Autodesk Inventor part; units mm, degrees
ref_plane "YZ Plane" through (0, 0, 0) normal (1, 0, 0) x (0, 1, 0)
ref_plane "XZ Plane" through (0, 0, 0) normal (0, 1, 0) x (-1, 0, 0)
ref_plane "XY Plane" through (0, 0, 0) normal (0, 0, 1) x (1, 0, 0)
sketch "Náčrt1" plane through (0, 0, 0) normal (0, 0, 1) x (1, 0, 0)
  line L0 (-4.9375, 15) -> (4.9375, 15)
  line L1 (4.9375, 15) -> (4.9375, -15)
  line L2 (4.9375, -15) -> (-4.9375, -15)
  line L3 (-4.9375, -15) -> (-4.9375, 15)
  line L4 (-4.9375, 15) -> (4.9375, -15) construction
  line L5 (4.9375, 15) -> (-4.9375, -15) construction
  circle A0 centre (0, 10.0625) radius 1.5
  circle A1 centre (0, -10.0625) radius 1.5
  line L6 (-4.9375, 0) -> (4.9375, 0)
  point P0 (0, 0)
  point P1 (0, 15)
  dimension "d0" = 30
  dimension "d1" = 9.875
  dimension "d2" = 3
  dimension "d4" = 4.9375
extrude "Vysunutí1" add sketch "Náčrt1" along normal blind 10
sketch "Náčrt2" plane through (4.9375, -15, 0) normal (1, 0, 0) x (0, 0, -1)
  line L0 (0, 0) -> (0, 30)
  line L1 (0, 10) -> (-3.3166, 10)
  arc A0 (-3.3166, 20) -> (-3.3166, 10) centre (0, 15) ccw
  line L2 (-3.3166, 20) -> (0, 20)
  line L3 (0, 9.875) -> (-3.3541, 9.875)
  arc A1 (-3.3541, 20.125) -> (-3.3541, 9.875) centre (0, 15) ccw
  line L4 (-3.3541, 20.125) -> (0, 20.125)
  line L5 (0, 30) -> (-10, 30)
  line L6 (0, 6.875) -> (-4.1533, 6.875) construction
  arc A2 (-4.1533, 23.125) -> (-4.1533, 6.875) centre (0, 15) ccw construction
  line L7 (-4.1533, 23.125) -> (0, 23.125) construction
  line L8 (0, 0) -> (-10, 0)
  line L9 (-7, 0) -> (-7, 9.1463)
  line L10 (-7, 9.1463) -> (-9, 13.4948)
  line L11 (-9, 16.5052) -> (-7, 20.8537)
  line L12 (-7, 20.8537) -> (-7, 30)
  line L13 (-9, 13.4948) -> (-9, 16.5052)
  line L14 (-10, 0) -> (-10, 30)
  point P0 (0, 15)
  point P1 (0, 9.875)
  point P2 (-9, 15)
  point P3 (-10, 15)
  dimension "d7" = 6
  dimension "d8" = 10
  dimension "d9" = 0.125
  dimension "d16" = 3
  dimension "d17" = 3
  dimension "d18" = 3
  dimension "d19" = 1
extrude "Vysunutí2" cut sketch "Náčrt2" against normal through all contours L3 A1 L4 L0 L2 A0 L1 | L8 L14 L5 L12 L11 L13 L10 L9 | L1 A0 L2 L0
fillet "Zaoblení1" radius 2 4 edges at (0, -1.5052, 9) (0, 1.5052, 9) (0, 5.8537, 7) (0, -5.8537, 7)
fillet "Zaoblení2" radius 0.25 20 edges at (0, -15, 7) (0, 15, 7) (4.9375, -5.8638, 7.0463) (4.9375, -3.6794, 8) (4.9375, -1.4951, 8.9537) (4.9375, 0, 9) (4.9375, 1.4951, 8.9537) (4.9375, 3.6794, 8) (4.9375, 5.8638, 7.0463) (4.9375, 10.6458, 7) (4.9375, -10.6458, 7) (-4.9375, -5.8638, 7.0463) (-4.9375, -3.6794, 8) (-4.9375, -1.4951, 8.9537) (-4.9375, 0, 9) (-4.9375, 1.4951, 8.9537) (-4.9375, 3.6794, 8) (-4.9375, 5.8638, 7.0463) (-4.9375, 10.6458, 7) (-4.9375, -10.6458, 7)
sketch "Náčrt3" plane through (0, 0, 0) normal (0, 0, -1) x (-1, 0, 0)
  line L0 (4.9375, -5.125) -> (-4.9375, -5.125)
  line L1 (-4.9375, -15) -> (-4.9375, -5.125)
  line L2 (4.9375, -15) -> (-4.9375, -15)
  line L3 (4.9375, -5.125) -> (4.9375, -15)
  circle A0 centre (0, -10.0625) radius 1.5
  line L4 (-4.9375, 5.125) -> (4.9375, 5.125)
  line L5 (4.9375, 15) -> (4.9375, 5.125)
  line L6 (-4.9375, 15) -> (4.9375, 15)
  line L7 (-4.9375, 5.125) -> (-4.9375, 15)
  circle A1 centre (0, 10.0625) radius 1.5
  point P0 (0, 0)
extrude "Vysunutí3" cut sketch "Náčrt3" against normal blind 1
chamfer "Zkosení1" distance 0.25 angle 45 6 edges at (4.9375, -5.125, 2.1771) (4.9375, 0, 6.125) (4.9375, 5.125, 2.1771) (-4.9375, -5.125, 2.1771) (-4.9375, 0, 6.125) (-4.9375, 5.125, 2.1771)
fillet "Zaoblení3" radius 0.5 8 edges at (4.8643, -14.9268, 6.9268) (4.9375, -15, 3.875) (-4.8643, -14.9268, 6.9268) (-4.9375, -15, 3.875) (-4.8643, 14.9268, 6.9268) (-4.9375, 15, 3.875) (4.8643, 14.9268, 6.9268) (4.9375, 15, 3.875)
sketch "Náčrt4" plane through (-4.6875, 6.2916, 7) normal (0, 0, 1) x (1, 0, 0)
  circle A0 centre (4.6875, 3.7709) radius 1.5
  point P0 (4.6875, -6.2916)
hole "Díra1" at (0, 10.0625, 7) direction (0, 0, -1) diameter 3.5 end through all countersink diameter 7 countersink angle 90
sketch "Náčrt5" plane through (-4.6875, -6.2916, 7) normal (0, 0, 1) x (1, 0, 0)
  circle A0 centre (4.6875, -3.7709) radius 1.5
  point P0 (4.6875, 6.2916)
hole "Díra2" at (0, -10.0625, 7) direction (0, 0, -1) diameter 3.5 end through all countersink diameter 7 countersink angle 90
properties part number "Objímka motoru pro plochu s držákem"
Verification items for the finished model (mm, model axes). A direction names the side the tool comes from. Coordinates: 2 decimals unless noted, no trailing zeros. Write each loop counter-clockwise with the first axis right and the second up, starting at its lowest first coordinate (ties: lowest second). Pieces come first, ordered by that corner, then holes. Notation, with made-up numbers: M 85.5,18 L 120.5,18 A24 ccw 120.5,38 Z; hole C 7,-24 d11. An arc over 180 degrees is marked long. Answer as a JSON object with one key per item and string values. Group by question number.
(1) Cross-section at A-A, the plane z = 3. State how many separate pieces and enclosed holes the cut face has, and give its area (3 significant figures).
(2) Release check for a two-part mould opening along Y. For faces 1 (the face through (-2, 10, 1)), 2 (the face through (0.07, -3.7, 7.99)), 3 (the face through (-4.814, -0.088, 6.251)) record: +Y half, -Y half, draft (parallel to the pull), parting line (faces both ways), or undercut.
(3) Cross-section at C-C, the plane x = -4. Record the cut outline in (y, z) (3 decimals), and give its area (3 significant figures).
(4) Tool access check on faces 4 (the face through (2.1, 13.3, 7)), 5 (the face through (2.1, -13.4, 7)), 6 (the face through (4.862, 3.675, 7.924)). Record the directions out of +Z, -Z, +X, -X, +Y, -Y that give a thin tool (end or side, any length) a straight path to the whole face; none if there is none.
(5) Gauge pin test, flat ends, axial feed: pin 1 (3 mm diameter, centred on x = 0, y = 10.06, fed in from +Z); pin 2 (3 mm diameter, centred on x = 0, y = -5, fed in from +Z). Record the tip position at first contact, or that the pin passes through.
(6) Material ranges on line 1 (Y direction, x = 0, z = 3.1) (1 decimal); line 2 (Y direction, x = 2.75, z = 2.5) (3 decimals); line 3 (Y direction, x = 1.5, z = 2.5) (3 decimals), recorded low to high.
Reply:
{
 "1": {"separate pieces": "2", "enclosed holes": "2", "area": "175 mm²"},
 "2": {"face 1": "draft", "face 2": "-Y half", "face 3": "undercut"},
 "3": {"outline": "M -15,1 L -5.125,1 L -5.125,3.354 A6.125 cw 5.125,3.354 L 5.125,1 L 15,1 L 15,6.75 A0.25 ccw 14.75,7 L 6.292,7 A2 cw 5.456,7.183 L 1.903,8.817 A2 ccw 1.067,9 L -1.067,9 A2 ccw -1.903,8.817 L -5.456,7.183 A2 cw -6.292,7 L -14.75,7 A0.25 ccw -15,6.75 Z", "area": "151 mm²"},
 "4": {"face 4": "+Z, +X, -X, +Y", "face 5": "+Z, +X, -X, -Y", "face 6": "+Z, +X, +Y"},
 "5": {"pin 1": "through", "pin 2": "z = 8.08"},
 "6": {"line 1": "-15 to -11.8, -8.3 to -5.1, 5.1 to 8.3, 11.8 to 15", "line 2": "-15 to -5.125, 5.125 to 15", "line 3": "-15 to -10.964, -9.161 to -5.125, 5.125 to 9.161, 10.964 to 15"}
}
